The listing builds one solid part. Answer for the finished solid, in the listing's coordinates (mm). Give positions to 0.01 mm unless a question says otherwise; leave off trailing zeros. Order: outer loops, then holes, each group sorted by start corner. A loop starts at its lowest first (then second) coordinate and runs counter-clockwise, first axis right, second up. Notation, with made-up numbers: M -25,16 L 7,16 A11 ccw 7,31 Z; hole C 15.5,4 d5. An arc over 180 degrees is marked long. Answer as a JSON object with one key per item and string values. Group by question number.
```python
from build123d import *

# Parameters (mm, degrees)
F0_R     = 3
F1_DEPTH = 12


with BuildPart() as f1:
    # F0 (on Front) → F1 (new body)
    with BuildSketch(Plane.XZ):
        Polygon((0, 55), (0, 0), (55, 0), align=None)
        with Locations((7, 7)):
            Circle(F0_R, mode=Mode.SUBTRACT)
        with Locations((38, 7)):
            Circle(F0_R, mode=Mode.SUBTRACT)
        with Locations((7, 38)):
            Circle(F0_R, mode=Mode.SUBTRACT)
    extrude(amount=-F1_DEPTH)


solid = f1.part
```
Item 1: Consider probe 1 along Z at (x, y) = (7, 6); probe 2 along Z at (x, y) = (9, 3.25); probe 3 along Z at (x, y) = (38, 7.5). Determine where each line is inside the solid, lowest interval first. Write a range as from..to.
Item 2: Section C-C (y = 1.5) is taken. Determine the outline of the cut face in (x, z).
Item 3: Flat-ended cylindrical pins translate along their axes: P1, Ø1, axis at x = 36, y = 5.5, coming from the +Z side; P2, Ø1, axis at x = 9, y = 6, coming from the +Z side; P3, Ø4, axis at y = 2.5, z = 25, coming from the +X side. Find the tip coordinate at first contact, or state that the pin passes through.
Item 4: Section B-B (z = 38) is taken. Determine the outline of the cut face in (x, y).
Item 5: Section A-A (x = 38) is taken. Determine the outline of the cut face in (y, z).
Item 6: Determine the mould class of faces 1 (the cylindrical face through (8.61, 5.92, 40.53)), 2 (the flat face through (27, 6, 0)), 3 (the flat face through (28, 6, 27)), 4 (the cylindrical face through (9.77, 5.92, 5.85)) for opening direction X: released by +X, released by -X, zero draft, split by the parting line, or undercut.
Item 7: Section D-D (x = 7) is taken. Determine the outline of the cut face in (y, z).
Values found:
{
 "1": {"probe 1": "z = 0..4, 10..35, 41..48", "probe 2": "z = 0..4.76, 9.24..35.76, 40.24..46", "probe 3": "z = 0..4, 10..17"},
 "2": {"outline": "M 0,0 L 55,0 L 0,55 Z; hole C 7,7 d6; hole C 7,38 d6; hole C 38,7 d6"},
 "3": {"P1": "stops at z = 19.5", "P2": "stops at z = 46.5", "P3": "stops at x = 32"},
 "4": {"outline": "M 0,0 L 4,0 L 4,12 L 0,12 Z; M 10,0 L 17,0 L 17,12 L 10,12 Z"},
 "5": {"outline": "M 0,0 L 12,0 L 12,4 L 0,4 Z; M 0,10 L 12,10 L 12,17 L 0,17 Z"},
 "6": {"face 1": "undercut", "face 2": "zero draft", "face 3": "released by +X", "face 4": "undercut"},
 "7": {"outline": "M 0,0 L 12,0 L 12,4 L 0,4 Z; M 0,10 L 12,10 L 12,35 L 0,35 Z; M 0,41 L 12,41 L 12,48 L 0,48 Z"}
}
